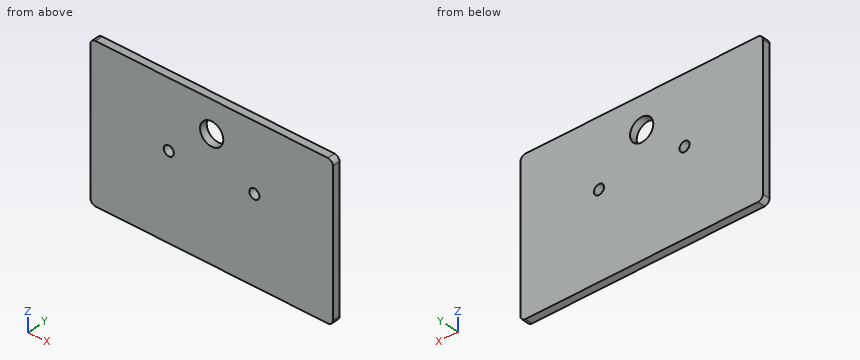
```python
from build123d import *

# Parameters (mm, degrees)
SKETCH1_W           = 72
SKETCH1_H           = 45
BOSS_EXTRUDE1_DEPTH = 2.25
FILLET2_R           = 1.5
FILLET3_R           = 1.5
SKETCH16_R          = 3.45
CUT_EXTRUDE1_DEPTH  = 10
SKETCH18_R          = 1.5
CUT_EXTRUDE2_DEPTH  = 10


with BuildPart() as part:
    # Sketch1 → Boss-Extrude1 (new body)
    with BuildSketch(Plane(origin=(0, 0, 0), x_dir=(1, 0, 0), z_dir=(0, 1, 0))):
        Rectangle(SKETCH1_W, SKETCH1_H)
    extrude(amount=BOSS_EXTRUDE1_DEPTH)

    # Fillet2
    fillet2_edges = [part.edges().sort_by_distance(p)[0] for p in [
        (-36, 1.125, -22.5),
    ]]
    fillet(fillet2_edges, radius=FILLET2_R)

    # Fillet3
    fillet3_edges = [part.edges().sort_by_distance(p)[0] for p in [
        (36, 1.125, 22.5),
        (-36, 1.125, 22.5),
        (36, 1.125, -22.5),
    ]]
    fillet(fillet3_edges, radius=FILLET3_R)

    # Sketch16 → Cut-Extrude1 (cut)
    with BuildSketch(Plane(origin=(0, 2.25, 0), x_dir=(1, 0, 0), z_dir=(0, 1, 0))):
        with Locations(Location((0, -13.097290255, 0), (0, 0, 270))):
            Circle(SKETCH16_R)
    extrude(amount=-CUT_EXTRUDE1_DEPTH, mode=Mode.SUBTRACT)

    # Sketch18 → Cut-Extrude2 (cut)
    with BuildSketch(Plane(origin=(0, 2.25, 0), x_dir=(1, 0, 0), z_dir=(0, 1, 0))):
        with Locations(Location((-12.734859634, -2.656879133, 0), (0, 0, 270))):
            Circle(SKETCH18_R)
        with Locations(Location((12.682272565, -2.656879133, 0), (0, 0, 270))):
            Circle(SKETCH18_R)
    extrude(amount=-CUT_EXTRUDE2_DEPTH, mode=Mode.SUBTRACT)


solid = part.part
```
For this review, take the finished solid that the model builds, in its own axes (mm). Round coordinates to 2 decimals unless told otherwise and drop trailing zeros. Write each loop counter-clockwise with the first axis right and the second up, starting at its lowest first coordinate (ties: lowest second). Pieces come first, ordered by that corner, then holes.
1) Take a section at A-A on x = 0. Give the boundary of the cut face in (y, z), then the cut area to 3 significant figures.
Answer below:
outline: (0, -22.5) - (2.25, -22.5) - (2.25, 9.65) - (0, 9.65) - close; (0, 16.55) - (2.25, 16.55) - (2.25, 22.5) - (0, 22.5) - close
area: 85.7 mm2
2) Take a section at B-B on z = 14. Give the boundary of the cut face in (x, y), then the cut area to 3 significant figures.
Answer below:
outline: (-36, 0) - (-3.33, 0) - (-3.33, 2.25) - (-36, 2.25) - close; (3.33, 0) - (36, 0) - (36, 2.25) - (3.33, 2.25) - close
area: 147 mm2
3) Take a section at C-C on y = 0.5. Give the boundary of the cut face in (x, z), then the cut area to 3 significant figures.
Answer below:
outline: (-36, -21) arc R1.5 ccw to (-34.5, -22.5) - (34.5, -22.5) arc R1.5 ccw to (36, -21) - (36, 21) arc R1.5 ccw to (34.5, 22.5) - (-34.5, 22.5) arc R1.5 ccw to (-36, 21) - close; hole circle Ø3 at (-12.73, 2.66); hole circle Ø6.9 at (0, 13.1); hole circle Ø3 at (12.68, 2.66)
area: 3,190 mm2
4) For line 1 along X through (y, z) = (0.4, 2); line 2 along X through (y, z) = (0.45, 3); line 3 along X through (y, z) = (0.8, 11.5), list the stretches that pass through material, from the lowest coordinate up.
Answer below:
line 1: x = -36 to -14.08, -11.39 to 11.33, 14.03 to 36
line 2: x = -36 to -14.2, -11.27 to 11.22, 14.14 to 36
line 3: x = -36 to -3.06, 3.06 to 36
